Part model, mm, in its own coordinate system. Face numbers are marked on the shaded views. A direction names the side the tool comes from. Coordinates: 2 decimals unless noted, no trailing zeros. Write each loop counter-clockwise with the first axis right and the second up, starting at its lowest first coordinate (ties: lowest second). Pieces come first, ordered by that corner, then holes. Notation, with made-up numbers: (44.25, 57) - (69.25, 57) arc R11 cw to (69.25, 69) - close; hole circle Ø3 at (-6, 13). An arc over 180 degrees is marked (long way). Use a Markdown table: item, result.
```python
from build123d import *

# Parameters (mm, degrees)
BOSS_EXTRUDE1_DEPTH     = 100
SHELL1_START            = 20
SHELL1_DEPTH            = 60
CUT_EXTRUDE5_DEPTH      = 700
CUT_EXTRUDE5_DEPTH_BACK = 1226.510966311
SKETCH3_R               = 2.5


# Read off the part's stored shape, not the designer's step: Shell1
with BuildPart() as part:
    # Sketch1 → Boss-Extrude1 (new body)
    with BuildSketch(Plane.XY):
        with BuildLine():
            Line((0, 0), (1000, 0))
            ThreePointArc((1000, 0), (1050, -50), (1000, -100))
            Line((1000, -100), (-150, -100))
            ThreePointArc((-150, -100), (-181.887821353, -75.531614088), (-166.506350946, -38.397459622))
            Line((-166.506350946, -38.397459622), (975, 620.651539379))
            ThreePointArc((975, 620.651539379), (1009.150635095, 611.500904284), (1000, 577.35026919))
            Line((1000, 577.35026919), (0, 0))
        make_face()
    extrude(amount=BOSS_EXTRUDE1_DEPTH)

    # Shell1 outline → Shell1 (cut)
    with BuildSketch(Plane.XY.offset(SHELL1_START)):
        with BuildLine():
            Line((-150, -80), (-150, -100))
            Line((-150, -100), (1000, -100))
            Line((1000, -100), (1000, -80))
            ThreePointArc((1000, -80), (1030, -50), (1000, -20))
            Line((1000, -20), (-74.641016151, -20))
            Line((-74.641016151, -20), (990, 594.670777265))
            ThreePointArc((990, 594.670777265), (991.830127019, 601.500904284), (985, 603.331031303))
            Line((985, 603.331031303), (975, 620.651539379))
            Line((975, 620.651539379), (-166.506350946, -38.397459622))
            Line((-166.506350946, -38.397459622), (-156.506350946, -55.717967697))
            ThreePointArc((-156.506350946, -55.717967697), (-162.569304827, -70.355233185), (-150, -80))
        make_face()
    extrude(amount=SHELL1_DEPTH, mode=Mode.SUBTRACT)

    # Sketch3 → Cut-Extrude5 (cut, two sides: drawn at the far end of the back side and taken through both)
    with BuildSketch(Plane(origin=(0, 0, 0), x_dir=(1, 0, 0), z_dir=(0, 1, 0)).offset(-CUT_EXTRUDE5_DEPTH_BACK)):
        with Locations(Location((200, -50, 0), (0, 0, 90))):
            Circle(SKETCH3_R)
        with Locations(Location((300, -50, 0), (0, 0, 90))):
            Circle(SKETCH3_R)
        with Locations(Location((400, -50, 0), (0, 0, 90))):
            Circle(SKETCH3_R)
        with Locations(Location((500, -50, 0), (0, 0, 90))):
            Circle(SKETCH3_R)
        with Locations(Location((600, -50, 0), (0, 0, 90))):
            Circle(SKETCH3_R)
        with Locations(Location((700, -50, 0), (0, 0, 90))):
            Circle(SKETCH3_R)
        with Locations(Location((800, -50, 0), (0, 0, 90))):
            Circle(SKETCH3_R)
        with Locations(Location((900, -50, 0), (0, 0, 90))):
            Circle(SKETCH3_R)
    extrude(amount=CUT_EXTRUDE5_DEPTH + CUT_EXTRUDE5_DEPTH_BACK, mode=Mode.SUBTRACT)


solid = part.part
```
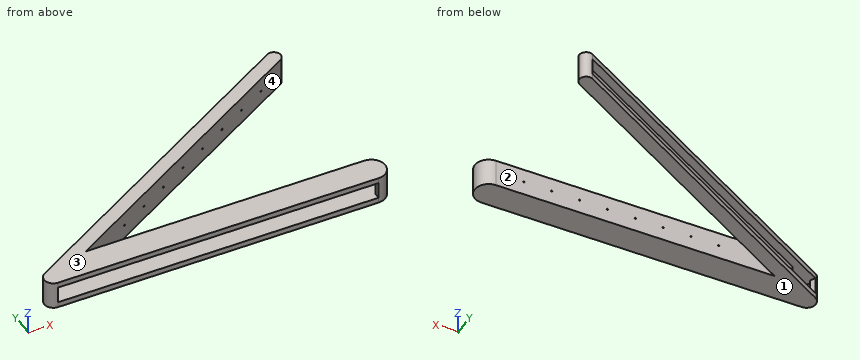
Item 1: Drop flat-ended pins along their axis: P1, Ø6, axis at x = 800, z = 50, coming from the +Y side; P2, Ø6.5, axis at x = 700, z = 50, coming from the +Y side; P3, Ø12, axis at x = 925.5, z = 74.5, coming from the -Y side; P4, Ø6.5, axis at x = 400, z = 50, coming from the +Y side. Give the stop position or say it passes through.
From the geometry:
| item | result |
|---|---|
| P1 | y = 486.71 |
| P2 | y = 429.12 |
| P3 | y = -100 |
| P4 | y = 255.91 |
Item 2: Band-saw the part on A-A, the plane x = 883. Give the cut face in (y, z), then the cut area to 3 significant figures.
From the geometry:
| item | result |
|---|---|
| outline | (-100, 0) - (0, 0) - (0, 100) - (-100, 100) - (-100, 80) - (-20, 80) - (-20, 20) - (-100, 20) - close; (509.8, 0) - (567.54, 0) - (567.54, 20) - (532.89, 20) - (532.89, 80) - (567.54, 80) - (567.54, 100) - (509.8, 100) - close |
| area | 8,900 mm^2 |
Item 3: Band-saw the part on B-B, the plane y = 14.5. Give the cut face in (x, z), then the cut area to 3 significant figures.
From the geometry:
| item | result |
|---|---|
| outline | (-74.89, 0) - (25.11, 0) - (25.11, 100) - (-74.89, 100) - (-74.89, 80) - (-14.89, 80) - (-14.89, 20) - (-74.89, 20) - close |
| area | 6,400 mm^2 |
Item 4: Which spindle directions (+Z, -Z, +X, -X, +Y, -Y) get a long thin tool onto all of the face, cutting with end or side? Do the marked faces 1 and 2. Say none if no direction does.
From the geometry:
| item | result |
|---|---|
| face 1 | -Z, +X, -X, +Y, -Y |
| face 2 | +Z, -Z, +X |
Item 5: Two-plate mould, pull along Y, no slides. Class the marked faces 3 and 4: pulls with the +Y half, pulls with the -Y half, needs draft (parallel to the pull), parting line crosses it, or undercut.
From the geometry:
| item | result |
|---|---|
| face 3 | needs draft |
| face 4 | undercut |
Item 6: Drill centre lines: probe 1 along Z at (x, y) = (900, -7); probe 2 along Z at (x, y) = (534.5, 335); probe 3 along Y at (x, z) = (777, 49). Where is each one in solid material? Low to high.
From the geometry:
| item | result |
|---|---|
| probe 1 | 0 to 47.5, 52.5 to 100 |
| probe 2 | 0 to 20, 80 to 100 |
| probe 3 | -20 to 0, 448.6 to 471.7 |
